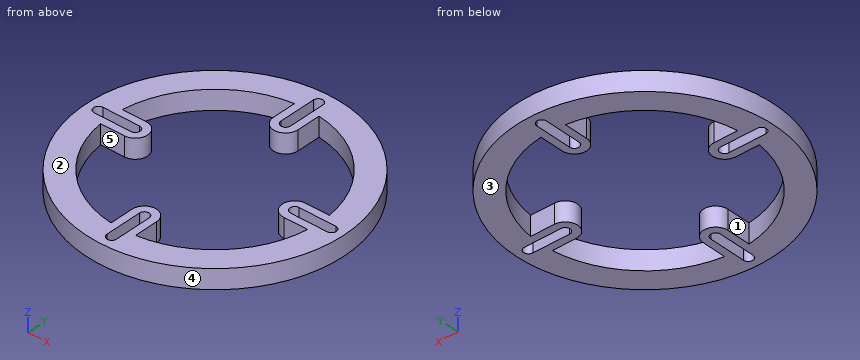
```python
from build123d import *

# Parameters (mm, degrees)
SKETCH2_R          = 53.34
SKETCH2_R_2        = 43.18
EXTRUDE3_DEPTH     = 8
EXTRUDE4_DEPTH     = 8
EXTRUDE5_DEPTH     = 8
CUT_EXTRUDE1_DEPTH = 9
CUT_EXTRUDE2_DEPTH = 9


with BuildPart() as part:
    # Sketch2 → Extrude3 (new body)
    with BuildSketch(Plane.XY):
        Circle(SKETCH2_R)
        Circle(SKETCH2_R_2, mode=Mode.SUBTRACT)
    extrude(amount=EXTRUDE3_DEPTH)

    # Sketch3 → Extrude4 (add)
    with BuildSketch(Plane.XY.offset(8)):
        with BuildLine():
            ThreePointArc((5.08, 48.26), (0, 43.18), (-5.08, 48.26))
            Line((-5.08, 48.26), (-5.08, 33.02))
            ThreePointArc((-5.08, 33.02), (0, 27.94), (5.08, 33.02))
            Line((5.08, 33.02), (5.08, 48.26))
        make_face()
    extrude4 = extrude(amount=-EXTRUDE4_DEPTH)

    # Mirror1: Extrude4 across plane
    add(extrude4.mirror(Plane.ZX))

    # Sketch4 → Extrude5 (add)
    with BuildSketch(Plane.XY.offset(8)):
        with BuildLine():
            ThreePointArc((-48.26, 5.08), (-43.18, 0), (-48.26, -5.08))
            Line((-48.26, -5.08), (-33.02, -5.08))
            ThreePointArc((-33.02, -5.08), (-27.94, 0), (-33.02, 5.08))
            Line((-33.02, 5.08), (-48.26, 5.08))
        make_face()
    extrude5 = extrude(amount=-EXTRUDE5_DEPTH)

    # Mirror2: Extrude5 across plane
    add(extrude5.mirror(Plane(origin=(0, 0, 0), x_dir=(0, 0, 1), z_dir=(1, 0, 0))))

    # Sketch5 → Cut-Extrude1 (cut, through all)
    with BuildSketch(Plane.XY.offset(8)):
        with BuildLine():
            Line((2, 33.02), (2, 48.26))
            ThreePointArc((2, 48.26), (0, 50.26), (-2, 48.26))
            Line((-2, 48.26), (-2, 33.02))
            ThreePointArc((-2, 33.02), (0, 31.02), (2, 33.02))
        make_face()
    cut_extrude1 = extrude(amount=-CUT_EXTRUDE1_DEPTH, mode=Mode.SUBTRACT)

    # Mirror3: Cut-Extrude1 across plane
    add(cut_extrude1.mirror(Plane.ZX), mode=Mode.SUBTRACT)

    # Sketch6 → Cut-Extrude2 (cut, through all)
    with BuildSketch(Plane.XY.offset(8)):
        with BuildLine():
            Line((-33.02, 2), (-48.26, 2))
            ThreePointArc((-48.26, 2), (-50.26, 0), (-48.26, -2))
            Line((-48.26, -2), (-33.02, -2))
            ThreePointArc((-33.02, -2), (-31.02, 0), (-33.02, 2))
        make_face()
    cut_extrude2 = extrude(amount=-CUT_EXTRUDE2_DEPTH, mode=Mode.SUBTRACT)

    # Mirror4: Cut-Extrude2 across plane
    add(cut_extrude2.mirror(Plane(origin=(0, 0, 0), x_dir=(0, 0, 1), z_dir=(1, 0, 0))), mode=Mode.SUBTRACT)


solid = part.part
```
Source: CAD feature listing. Evaluate the final solid. Frame: model axes, mm. Face numbers are marked on the shaded views. A direction names the side the tool comes from. Give positions to 0.01 mm unless a question says otherwise; leave off trailing zeros. Write each loop counter-clockwise with the first axis right and the second up, starting at its lowest first coordinate (ties: lowest second). Pieces come first, ordered by that corner, then holes. Notation, with made-up numbers: (40.5, 54.5) - (94.5, 54.5) arc R22 cw to (94.5, 91.5) - close; hole circle Ø10 at (62, 11.25). An arc over 180 degrees is marked (long way). One line per item, written item: value. Start each with the question number.
Q1. Set-up query: the marked faces 1 and 2. Return all of +Z, -Z, +X, -X, +Y, -Y with unobstructed straight access to the full face (end or side cutting, diameter ignored); none if empty.
Q2. Material intervals for probe 1 along X at (y, z) = (-31.5, 4.75); probe 2 along Y at (x, z) = (-34.5, 7.25); probe 3 along Y at (x, z) = (40, 4.75), sorted ascending. Write a range as from..to.
Q3. Draft query along X for the marked faces 3, 4 and 5. Return one class per face: +X half, -X half, draft (parallel to the pull), parting line (faces both ways), or undercut.
Q4. First-contact query: pin 1 Ø4 at (x, z) = (-44, 3) entering from +Y; pin 2 Ø2.5 at (x, z) = (41, 5.5) entering from -Y; pin 3 Ø2.5 at (y, z) = (36.5, 4) entering from -X. Flat tips, straight axial feed; report the tip coordinate or a pass-through.
Q5. Section query D-D, the plane y = 26. Return the cut outline in (x, z).
Q6. Section query A-A, the plane z = 4. Count the separate pieces of the cut face and the enclosed holes in it, then the cut area to 3 significant figures.
Q7. Section query B-B, the plane x = 0. Return the cut outline in (y, z).
Answer:
1. face 1: +Z, -Z
1. face 2: +Z, +X, -X, +Y, -Y
2. probe 1: x = -43.05..-29.53, -4.85..-1.3, 1.3..4.85, 29.53..43.05
2. probe 2: y = -40.68..-25.97, -5.08..-2, 2..5.08, 25.97..40.68
2. probe 3: y = -35.29..-16.26, -5.08..-2, 2..5.08, 16.26..35.29
3. face 3: draft
3. face 4: parting line
3. face 5: undercut
4. pin 1: stops at y = 32.88
4. pin 2: stops at y = -35.57
4. pin 3: stops at x = -40.03
5. outline: (-46.57, 0) - (-34.47, 0) - (-34.47, 8) - (-46.57, 8) - close; (34.47, 0) - (46.57, 0) - (46.57, 8) - (34.47, 8) - close
6. separate pieces: 1
6. enclosed holes: 5
6. area: 3,360 mm2
7. outline: (-53.34, 0) - (-50.26, 0) - (-50.26, 8) - (-53.34, 8) - close; (-31.02, 0) - (-27.94, 0) - (-27.94, 8) - (-31.02, 8) - close; (27.94, 0) - (31.02, 0) - (31.02, 8) - (27.94, 8) - close; (50.26, 0) - (53.34, 0) - (53.34, 8) - (50.26, 8) - close
